Input: part model. Units: mm. Frame: model coordinates. A direction names the side the tool comes from. Give positions to 0.01 mm unless a question says otherwise; leave off trailing zeros. Write each loop counter-clockwise with the first axis right and the second up, starting at its lowest first coordinate (ties: lowest second). Pieces come first, ordered by that corner, then holes. Notation, with made-up numbers: (-11.5, 49) -> (-0.5, 49) arc R32 cw to (-0.5, 87) -> close; hole circle Ø5 at (43, 24.25). An arc over 180 degrees is marked (long way). Return JSON: item names as keys, results as strings. Group by question number.
Item 1: Section C-C, the plane z = 23.5. Return loops of the section in (x, y), then the cut area to 3 significant figures.
Item 2: Section A-A, the plane z = 11. Return loops of the section in (x, y), then the cut area to 3 significant figures.
Item 3: Section D-D, the plane x = -22. Return loops of the section in (y, z).
Item 4: Pin query (flat end, axial travel): P1, Ø1.5, axis at y = 16, z = 18.5, coming from the -X side; P2, Ø6, axis at x = 17, y = -12, coming from the +Z side; P3, Ø8, axis at x = 20, z = -20, coming from the +Y side; P4, Ø15.5, axis at x = 24, y = -11.5, coming from the -Z side. Return the tip coordinate at first contact, or that it passes through.
Item 5: Mould query, pull axis Y, two halves, no side actions, for faces 4 (the face through (0, 33, 0)), 5 (the face through (0, 19, -25)), 6 (the face through (0, -30, 0)), 7 (the face through (-16, -17, 2.5)). Classes: released by +Y, released by -Y, zero draft, split by the parting line, or undercut.
Item 6: Section B-B, the plane y = 0. Return loops of the section in (x, z), then the cut area to 3 significant figures.
Item 7: Set-up query: faces 1 (the face through (16, -25, -16)), 2 (the face through (11.087, 15.559, -27.535)), 3 (the face through (-16, -17, -2.5)). Return all of +Z, -Z, +X, -X, +Y, -Y with unobstructed straight access to the full face (end or side cutting, diameter ignored); none if empty.
Item 8: Line query: line 1 (X direction, y = -28.2, z = 20); line 2 (Z direction, x = -5.5, y = 20). Output: solid intervals per line, ascending. Write a range as [from, to].
from build123d import *

# Parameters (mm, degrees)
SKETCH_2_R               = 11
EXTRUDE_2_DEPTH          = 30
SKETCH_2_6_R             = 4
EXTRUDE_3_DEPTH          = 2.5
EXTRUDE_START            = 15
EXTRUDE_4_DEPTH          = 5
EXTRUDE_START_2          = -30
EXTRUDE_5_DEPTH          = 5
SKETCH_4_R               = 4.5
CUT_EXTRUDE_1_DEPTH      = 72.860976893
MIRROR_2_COPY_1_SKETCH_R = 4.5
MIRROR_2_COPY_1_DEPTH    = 72.860976893
FILLET_1_R               = 10


with BuildPart() as part:
    # Эскиз2 → Бобышка-Вытянуть2 (new, symmetric)
    with BuildSketch(Plane.XY):
        with BuildLine():
            Line((-6.5, -13.518505835), (-6.5, -25))
            Line((-6.5, -25), (-30, -25))
            Line((-30, -25), (-30, -30))
            Line((-30, -30), (30, -30))
            Line((30, -30), (30, -25))
            Line((30, -25), (6.5, -25))
            Line((6.5, -25), (6.5, -13.518505835))
            ThreePointArc((6.5, -13.518505835), (0, 15), (-6.5, -13.518505835))
        make_face()
        Circle(SKETCH_2_R, mode=Mode.SUBTRACT)
    extrude(amount=EXTRUDE_2_DEPTH, both=True)

    # Эскиз2<6> → Бобышка-Вытянуть3 (add, symmetric)
    with BuildSketch(Plane.XY):
        with BuildLine():
            ThreePointArc((-14.4, 4.2), (-9, 12), (0, 15))
            ThreePointArc((0, 15), (9, 12), (14.4, 4.2))
            Line((14.4, 4.2), (7.68, 27.24))
            ThreePointArc((7.68, 27.24), (0, 33), (-7.68, 27.24))
            Line((-7.68, 27.24), (-14.4, 4.2))
        make_face()
        with Locations((0, 25)):
            Circle(SKETCH_2_6_R, mode=Mode.SUBTRACT)
        with BuildLine():
            ThreePointArc((-6.5, -13.518505835), (-10.865729218, -10.340982959), (-13.823441352, -5.823441352))
            Line((-13.823441352, -5.823441352), (-30, -22))
            Line((-30, -22), (-30, -25))
            Line((-30, -25), (-6.5, -25))
            Line((-6.5, -25), (-6.5, -13.518505835))
        make_face()
        with BuildLine():
            Line((30, -22), (13.823441352, -5.823441352))
            ThreePointArc((13.823441352, -5.823441352), (10.865729218, -10.340982959), (6.5, -13.518505835))
            Line((6.5, -13.518505835), (6.5, -25))
            Line((6.5, -25), (30, -25))
            Line((30, -25), (30, -22))
        make_face()
    extrude(amount=EXTRUDE_3_DEPTH, both=True)

    # Эскиз2<8> → Бобышка-Вытянуть4 (add)
    with BuildSketch(Plane.XY.offset(EXTRUDE_START)):
        with BuildLine():
            ThreePointArc((-14.4, 4.2), (-9, 12), (0, 15))
            ThreePointArc((0, 15), (9, 12), (14.4, 4.2))
            Line((14.4, 4.2), (7.68, 27.24))
            ThreePointArc((7.68, 27.24), (0, 33), (-7.68, 27.24))
            Line((-7.68, 27.24), (-14.4, 4.2))
        make_face()
        with BuildLine():
            ThreePointArc((4, 25), (2.828427125, 22.171572875), (0, 21))
            ThreePointArc((0, 21), (-2.828427125, 27.828427125), (4, 25))
        make_face(mode=Mode.SUBTRACT)
    extrude(amount=EXTRUDE_4_DEPTH)

    # Эскиз2<9> → Бобышка-Вытянуть5 (add)
    with BuildSketch(Plane.XY.offset(EXTRUDE_START_2)):
        with BuildLine():
            ThreePointArc((-14.4, 4.2), (-9, 12), (0, 15))
            ThreePointArc((0, 15), (9, 12), (14.4, 4.2))
            Line((14.4, 4.2), (7.68, 27.24))
            ThreePointArc((7.68, 27.24), (0, 33), (-7.68, 27.24))
            Line((-7.68, 27.24), (-14.4, 4.2))
        make_face()
        with BuildLine():
            ThreePointArc((4, 25), (2.828427125, 22.171572875), (0, 21))
            ThreePointArc((0, 21), (-2.828427125, 27.828427125), (4, 25))
        make_face(mode=Mode.SUBTRACT)
    extrude(amount=EXTRUDE_5_DEPTH)

    # Эскиз4 → Вырез-Вытянуть1 (cut, through all)
    with BuildSketch(Plane(origin=(0, -25, 0), x_dir=(1, 0, 0), z_dir=(0, 1, 0))):
        with Locations(Location((20, 20, 0), (0, 0, 270))):
            Circle(SKETCH_4_R)
    cut_extrude_1 = extrude(amount=-CUT_EXTRUDE_1_DEPTH, mode=Mode.SUBTRACT)

    # Зеркальное отражение1: Вырез-Вытянуть1 across plane
    add(cut_extrude_1.mirror(Plane.XY), mode=Mode.SUBTRACT)

    # Зеркальное отражение2: Вырез-Вытянуть1 across plane
    add(cut_extrude_1.mirror(Plane(origin=(0, 0, 0), x_dir=(0, 0, 1), z_dir=(1, 0, 0))), mode=Mode.SUBTRACT)

    # Зеркальное отражение2 copy 1 sketch → Зеркальное отражение2 copy 1 (cut, through all)
    with BuildSketch(Plane(origin=(0, -25, 0), x_dir=(-1, 0, 0), z_dir=(0, 1, 0))):
        with Locations(Location((20, 20, 0), (0, 0, 270))):
            Circle(MIRROR_2_COPY_1_SKETCH_R)
    extrude(amount=-MIRROR_2_COPY_1_DEPTH, mode=Mode.SUBTRACT)

    # Скругление1
    fillet_1_edges = [part.edges().sort_by_distance(p)[0] for p in [
        (30, -27.5, -30),
        (-30, -27.5, -30),
        (-30, -27.5, 30),
        (30, -27.5, 30),
    ]]
    fillet(fillet_1_edges, radius=FILLET_1_R)


solid = part.part
Answer below:
{
 "1": {"outline": "(-29.37, -30) -> (-22.83, -30) -> (-22.83, -25) -> (-29.37, -25) -> close; (-17.17, -30) -> (17.17, -30) -> (17.17, -25) -> (6.5, -25) -> (6.5, -13.52) arc R15 ccw (long way) to (-6.5, -13.52) -> (-6.5, -25) -> (-17.17, -25) -> close; (22.83, -30) -> (29.37, -30) -> (29.37, -25) -> (22.83, -25) -> close; hole circle Ø22 at (0, 0)", "area": "700 mm2"},
 "2": {"outline": "(-30, -30) -> (30, -30) -> (30, -25) -> (6.5, -25) -> (6.5, -13.52) arc R15 ccw (long way) to (-6.5, -13.52) -> (-6.5, -25) -> (-30, -25) -> close; hole circle Ø22 at (0, 0)", "area": "763 mm2"},
 "3": {"outline": "(-30, -29.8) -> (-25, -29.8) -> (-25, -24.03) -> (-30, -24.03) -> close; (-30, -15.97) -> (-25, -15.97) -> (-25, -2.5) -> (-14, -2.5) -> (-14, 2.5) -> (-25, 2.5) -> (-25, 15.97) -> (-30, 15.97) -> close; (-30, 24.03) -> (-25, 24.03) -> (-25, 29.8) -> (-30, 29.8) -> close"},
 "4": {"P1": "stops at x = -11.18", "P2": "stops at z = 2.5", "P3": "passes through", "P4": "stops at z = -2.5"},
 "5": {"face 4": "released by +Y", "face 5": "zero draft", "face 6": "released by -Y", "face 7": "undercut"},
 "6": {"outline": "(-15, -30) -> (-11, -30) -> (-11, 30) -> (-15, 30) -> close; (11, -30) -> (15, -30) -> (15, 30) -> (11, 30) -> close", "area": "480 mm2"},
 "7": {"face 1": "-Z, +X", "face 2": "+Z, -Z, +X, +Y", "face 3": "-Z, -X"},
 "8": {"line 1": "x = [-30, -24.5], [-15.5, 15.5], [24.5, 30]", "line 2": "z = [-30, -25], [-2.5, 2.5], [15, 20]"}
}
